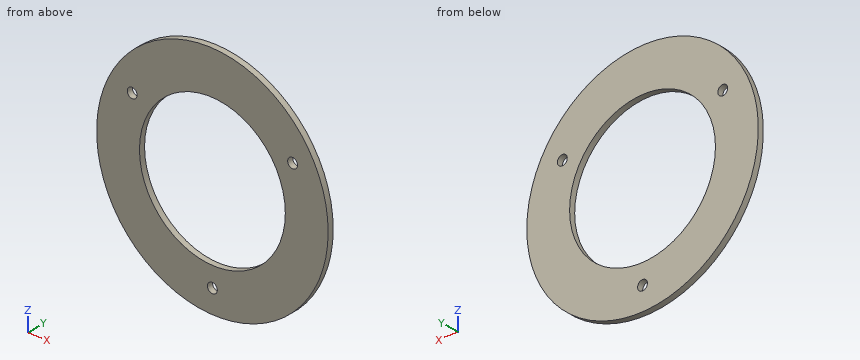
```python
from build123d import *

# Parameters (mm, degrees)
SKETCH1_R           = 63.5
BOSS_EXTRUDE1_DEPTH = 3.18
SKETCH2_R           = 40.005
CUT_EXTRUDE1_DEPTH  = 3.18
CIRPATTERN1_COUNT   = 3


with BuildPart() as part:
    # Sketch1 → Boss-Extrude1 (new body)
    with BuildSketch(Plane(origin=(0, 0, 0), x_dir=(1, 0, 0), z_dir=(0, 1, 0))):
        Circle(SKETCH1_R)
    extrude(amount=BOSS_EXTRUDE1_DEPTH)

    # Sketch2 → Cut-Extrude1 (cut)
    with BuildSketch(Plane(origin=(0, 3.18, 0), x_dir=(1, 0, 0), z_dir=(0, 1, 0))):
        Circle(SKETCH2_R)
    extrude(amount=-CUT_EXTRUDE1_DEPTH, mode=Mode.SUBTRACT)

    # Sketch7 → Hole for #8 300® SC Nuts (SP)1 (revolve, cut)
    with BuildSketch(Plane(origin=(0, 3.18, -50.8), x_dir=(0, 0, 1), z_dir=(1, 0, 0))):
        Polygon((0, 0), (0, 21.375388061), (2.7051, 19.75), (2.7051, 0), align=None)
    hole_for_8_300_sc_nuts_sp_1 = revolve(axis=Axis((0, 9.53, -50.8), (0, -1, 0)), mode=Mode.SUBTRACT)

    # CirPattern1: Hole for #8 300® SC Nuts (SP)1 ×3 about axis
    cirpattern1_axis = Axis((0, 0, 0), (0, 1, 0))
    for i in range(1, CIRPATTERN1_COUNT):
        add(hole_for_8_300_sc_nuts_sp_1.rotate(cirpattern1_axis, i * 360 / CIRPATTERN1_COUNT), mode=Mode.SUBTRACT)


solid = part.part
```
CAD build for the part. Positions are in the model's coordinates, mm. Give positions to 0.01 mm unless a question says otherwise; leave off trailing zeros. Loops run counter-clockwise (first coordinate to the right, second up) from the corner with the lowest first, then second, coordinate; pieces in that order, holes last. Notation, with made-up numbers: M -4,-26 L 11,-26 A11 ccw 11,-13 Z; hole C 15,-8.5 d2. An arc over 180 degrees is marked long. Use one line per item in the form item = value.
Item 1: Flat gauge pins, fed straight in: pin 1 (6 mm diameter, centred on x = -45, z = 48.5, fed in from -Y); pin 2 (3 mm diameter, centred on x = 43.99, z = 25.4, fed in from +Y); pin 3 (1 mm diameter, centred on y = 0.5, z = -10, fed in from +X). Where does each tip first touch, or does it go through?
Determined:
pin_1 = 0
pin_2 = through
pin_3 = 62.79
Item 2: Slice it at A-A (z = -50.8). List the corners of the cut face in (x, y).
Determined:
outline = M -38.1,0 L -2.71,0 L -2.71,3.18 L -38.1,3.18 Z; M 2.71,0 L 38.1,0 L 38.1,3.18 L 2.71,3.18 Z
Item 3: Slice it at B-B (x = 0). List the corners of the cut face in (y, z) (3 decimals).
Determined:
outline = M 0,-63.5 L 3.18,-63.5 L 3.18,-53.505 L 0,-53.505 Z; M 0,-48.095 L 3.18,-48.095 L 3.18,-40.005 L 0,-40.005 Z; M 0,40.005 L 3.18,40.005 L 3.18,63.5 L 0,63.5 Z
Item 4: Slice it at C-C (x = -19.5). List the corners of the cut face in (y, z).
Determined:
outline = M 0,-60.43 L 3.18,-60.43 L 3.18,-34.93 L 0,-34.93 Z; M 0,34.93 L 3.18,34.93 L 3.18,60.43 L 0,60.43 Z
Item 5: Drill centre lines: probe 1 along Z at (x, y) = (0, 0.75) (3 decimals); probe 2 along X at (y, z) = (1.2, 25.4); probe 3 along Z at (x, y) = (-32, 1.6). Where is each one in solid material? Low to high. Write a range as from..to.
Determined:
probe_1 = -63.5..-53.505, -48.095..-40.005, 40.005..63.5
probe_2 = -58.2..-46.7, -41.29..-30.91, 30.91..41.29, 46.7..58.2
probe_3 = -54.85..-24.01, 24.01..54.85
Item 6: Slice it at D-D (y = 1.1). List the corners of the cut face in (x, z) (3 decimals).
Determined:
outline = C 0,0 d127; hole C -43.994,25.4 d5.41; hole C 0,0 d80.01; hole C 0,-50.8 d5.41; hole C 43.994,25.4 d5.41
